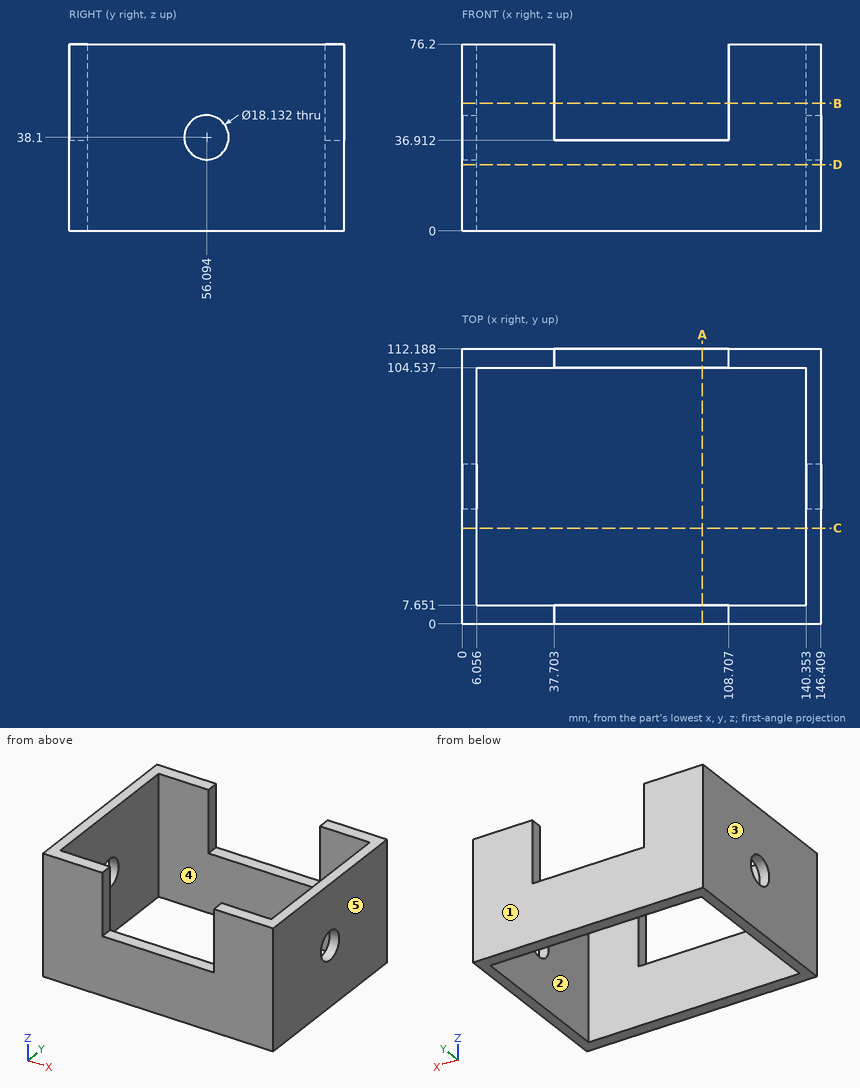
Design review of the part shown in the three views and the two pictorial views. Dimensions are in mm from the part's minimum x, y and z. A direction names the side the tool comes from. Give positions to 0.01 mm unless a question says otherwise; leave off trailing zeros. Loops run counter-clockwise (first coordinate to the right, second up) from the corner with the lowest first, then second, coordinate; pieces in that order, holes last. Notation, with made-up numbers: (47, 60) -> (63, 60) arc R22 cw to (63, 93) -> close; hole circle Ø5 at (42, 30). An arc over 180 degrees is marked (long way). Put each result on its own line as item: value. Start each with the question number.
1. We need section D-D on z = 27. State the section outline as (x, y) points.
2. Mouldability with a two-part tool opening along Y and no side actions: class the marked faces 1, 2 and 3 as released by +Y, released by -Y, zero draft, split by the parting line, or undercut.
3. Clearance check with flat-ended pins moving along their axes: P1, Ø6, axis at x = 88.5, y = 107.5, coming from the +Z side; P2, Ø11, axis at y = 56.09, z = 38.1, coming from the +X side. State where each tip first meets the part, or that it passes through.
4. For the marked faces 4 and 5, list the 3-axis set-ups (+Z, -Z, +X, -X, +Y, -Y) from which the entire face can be reached by the end or side of a thin tool; tool diameter is ignored.
5. We need section A-A on x = 98. State the section outline as (y, z) points.
6. We need section B-B on z = 52. State the section outline as (x, y) points.
7. We need section C-C on y = 39. State the section outline as (x, z) points, then the cut area to 3 significant figures.
8. Wall thickness on probe 1 along X at (y, z) = (62, 63); probe 2 along Y at (x, z) = (107.5, 31.5); probe 3 along Y at (x, z) = (143, 38): over which ranges is each line inside the solid? List them lowest first.
Determined:
1. outline: (0, 0) -> (146.41, 0) -> (146.41, 112.19) -> (0, 112.19) -> close; hole (6.06, 7.65) -> (140.35, 7.65) -> (140.35, 104.54) -> (6.06, 104.54) -> close
2. face 1: released by +Y
2. face 2: undercut
2. face 3: zero draft
3. P1: z = 36.91
3. P2: through
4. face 4: +Z, -Z
4. face 5: +Z, -Z, +X, +Y, -Y
5. outline: (0, 0) -> (7.65, 0) -> (7.65, 36.91) -> (0, 36.91) -> close; (104.54, 0) -> (112.19, 0) -> (112.19, 36.91) -> (104.54, 36.91) -> close
6. outline: (0, 0) -> (37.7, 0) -> (37.7, 7.65) -> (6.06, 7.65) -> (6.06, 104.54) -> (37.7, 104.54) -> (37.7, 112.19) -> (0, 112.19) -> close; (108.71, 0) -> (146.41, 0) -> (146.41, 112.19) -> (108.71, 112.19) -> (108.71, 104.54) -> (140.35, 104.54) -> (140.35, 7.65) -> (108.71, 7.65) -> close
7. outline: (0, 0) -> (6.06, 0) -> (6.06, 76.2) -> (0, 76.2) -> close; (140.35, 0) -> (146.41, 0) -> (146.41, 76.2) -> (140.35, 76.2) -> close
7. area: 923 mm^2
8. probe 1: 0 to 6.06, 140.35 to 146.41
8. probe 2: 0 to 7.65, 104.54 to 112.19
8. probe 3: 0 to 47.03, 65.16 to 112.19
